Geometry: final body of the model. Coordinates: model frame, mm. Face numbers are marked on the shaded views. A direction names the side the tool comes from. Round coordinates to 2 decimals unless told otherwise and drop trailing zeros. Order: outer loops, then holes, each group sorted by start corner. A loop starts at its lowest first (then second) coordinate and runs counter-clockwise, first axis right, second up. Notation, with made-up numbers: (35.5, 32.25) - (64.5, 32.25) arc R23 ccw to (64.5, 63.25) - close; hole circle Ø9 at (-22.75, 68.5). An arc over 180 degrees is marked (long way). Put each result on its own line as item: value. Start each with the question number.
(1) Section B-B (y = 2.2). Output: boundary loops of the cut face in (x, z).
(2) Material intervals for L1, parallel to X at y = 2.35, z = 6; L2, parallel to X at y = 0.9, z = 6; L3, parallel to Z at x = 1, y = 2.1, sorted ascending. Write a range as [from, to].
(3) Pin query (flat end, axial travel): P1, Ø6, axis at x = -1.5, z = 1, coming from the +Y side; P2, Ø0.5, axis at y = 1.5, z = 6.5, coming from the +X side; P3, Ø2.5, axis at x = 1.25, z = 6, coming from the -Y side. Return the tip coordinate at first contact, or that it passes through.
(4) Access query for the marked faces 1, 2, 3, 4 and 5. Directions: +Z, -Z, +X, -X, +Y, -Y. A direction counts if a zero-diameter tool reaches every point of the face in a straight line with its end or side. Return the directions, or none.
(5) Section C-C (z = 6). Output: boundary loops of the cut face in (x, y).
(6) Pull-direction query (X, two-part tool) for the marked faces 6, 7 and 8; classes: released by +X, released by -X, zero draft, split by the parting line, or undercut.
(7) Section D-D (z = 2.5). Output: boundary loops of the cut face in (x, y).
(8) Section A-A (x = 1.25). Output: boundary loops of the cut face in (y, z).
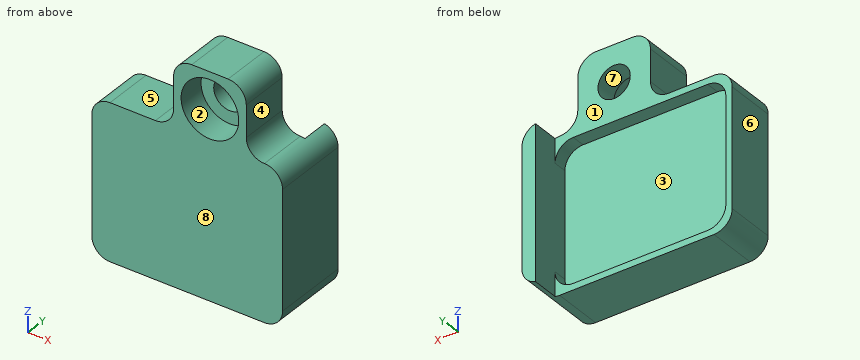
from build123d import *

# Parameters (mm, degrees)
SKETCH1_W                                      = 10.5
SKETCH1_H                                      = 8.5
EXTRUDE1_DEPTH                                 = 4.25
SKETCH3_W                                      = 9.75
SKETCH3_H                                      = 8.5
EXTRUDE4_DEPTH                                 = 1.5
SKETCH4_W                                      = 9.4
SKETCH4_H                                      = 7.8
EXTRUDE5_DEPTH                                 = 0.75
SKETCH5_W                                      = 4
SKETCH5_H                                      = 2.75
EXTRUDE6_DEPTH                                 = 3.75
CBORE_FOR_0_SOCKET_HEAD_CAP_SCREW1_D           = 1.778
CBORE_FOR_0_SOCKET_HEAD_CAP_SCREW1_CBORE_D     = 3.175
CBORE_FOR_0_SOCKET_HEAD_CAP_SCREW1_CBORE_DEPTH = 1.524
FILLET1_R                                      = 1


with BuildPart() as part:
    # Sketch1 → Extrude1 (new body)
    with BuildSketch(Plane(origin=(0, 0, 0), x_dir=(1, 0, 0), z_dir=(0, 1, 0))):
        Rectangle(SKETCH1_W, SKETCH1_H)
    extrude(amount=EXTRUDE1_DEPTH)

    # Sketch3 → Extrude4 (cut)
    with BuildSketch(Plane(origin=(0, 4.25, 0), x_dir=(1, 0, 0), z_dir=(0, 1, 0))):
        with Locations((-0.375, 0)):
            Rectangle(SKETCH3_W, SKETCH3_H)
    extrude(amount=-EXTRUDE4_DEPTH, mode=Mode.SUBTRACT)

    # Sketch4 → Extrude5 (cut)
    with BuildSketch(Plane(origin=(0, 2.75, 0), x_dir=(1, 0, 0), z_dir=(0, 1, 0))):
        with Locations((-0.2, 0)):
            Rectangle(SKETCH4_W, SKETCH4_H)
    extrude(amount=-EXTRUDE5_DEPTH, mode=Mode.SUBTRACT)

    # Sketch5 → Extrude6 (add)
    with BuildSketch(Plane.XY.offset(4.25)):
        with Locations((1.25, 1.375)):
            Rectangle(SKETCH5_W, SKETCH5_H)
    extrude(amount=EXTRUDE6_DEPTH)

    # CBORE for #0 Socket Head Cap Screw1 (through all)
    with Locations(Plane(origin=(1.25, 0, 6), x_dir=(0, 0, -1), z_dir=(0, -1, 0))):
        with Locations((0, 0)):
            CounterBoreHole(CBORE_FOR_0_SOCKET_HEAD_CAP_SCREW1_D / 2, CBORE_FOR_0_SOCKET_HEAD_CAP_SCREW1_CBORE_D / 2, CBORE_FOR_0_SOCKET_HEAD_CAP_SCREW1_CBORE_DEPTH)

    # Fillet1
    # the kernel refuses this fillet: 1 mm, written as the material it adds along each edge
    with BuildSketch(Plane(origin=(3.25, 2.75, 4.25), x_dir=(0, 0, 1), z_dir=(0, -1, 0))) as fillet1_piece_1:
        with BuildLine():
            CenterArc((FILLET1_R, -FILLET1_R), FILLET1_R, 90, 90)
            Line((0, -FILLET1_R), (0, 0))
            Line((0, 0), (FILLET1_R, 0))
        make_face()
    extrude(amount=2.75)
    with BuildSketch(Plane(origin=(-0.75, 0, 4.25), x_dir=(-1, 0, 0), z_dir=(0, 1, 0))) as fillet1_piece_2:
        with BuildLine():
            CenterArc((FILLET1_R, FILLET1_R), FILLET1_R, 180, 90)
            Line((0, FILLET1_R), (0, 0))
            Line((0, 0), (FILLET1_R, 0))
        make_face()
    extrude(amount=2.75)
    with BuildSketch(Plane(origin=(4.5, 2.75, -3.9), x_dir=(0, 0, 1), z_dir=(0, -1, 0)), Plane(origin=(-4.9, 2.75, -3.9), x_dir=(1, 0, 0), z_dir=(0, -1, 0)), Plane(origin=(-4.9, 2.75, 3.9), x_dir=(0, 0, -1), z_dir=(0, -1, 0))) as fillet1_piece_3:
        with BuildLine():
            CenterArc((FILLET1_R, FILLET1_R), FILLET1_R, 180, 90)
            Line((0, FILLET1_R), (0, 0))
            Line((0, 0), (FILLET1_R, 0))
        make_face()
    extrude(amount=0.75)
    with BuildSketch(Plane(origin=(4.5, 2.75, 3.9), x_dir=(0, 0, -1), z_dir=(0, -1, 0))) as fillet1_piece_4:
        with BuildLine():
            CenterArc((FILLET1_R, -FILLET1_R), FILLET1_R, 90, 90)
            Line((0, -FILLET1_R), (0, 0))
            Line((0, 0), (FILLET1_R, 0))
        make_face()
    extrude(amount=0.75)
    # the kernel refuses this fillet: 1 mm, written as the material it takes off along each edge
    with BuildSketch(Plane(origin=(5.25, -2.5, -4.25), x_dir=(-1, 0, 0), z_dir=(0, 1, 0)), Plane(origin=(5.25, -2.5, 4.25), x_dir=(0, 0, -1), z_dir=(0, 1, 0))) as fillet1_2_piece_1:
        with BuildLine():
            CenterArc((FILLET1_R, FILLET1_R), FILLET1_R, 180, 90)
            Line((0, FILLET1_R), (0, 0))
            Line((0, 0), (FILLET1_R, 0))
        make_face()
    extrude(amount=9.25, mode=Mode.SUBTRACT)
    with BuildSketch(Plane(origin=(3.25, 5.25, 8), x_dir=(0, 0, -1), z_dir=(0, -1, 0))) as fillet1_2_piece_2:
        with BuildLine():
            CenterArc((FILLET1_R, -FILLET1_R), FILLET1_R, 90, 90)
            Line((0, -FILLET1_R), (0, 0))
            Line((0, 0), (FILLET1_R, 0))
        make_face()
    extrude(amount=7.75, mode=Mode.SUBTRACT)
    with BuildSketch(Plane(origin=(-0.75, -2.5, 8), x_dir=(1, 0, 0), z_dir=(0, 1, 0)), Plane(origin=(-5.25, -2.5, -4.25), x_dir=(0, 0, 1), z_dir=(0, 1, 0)), Plane(origin=(-5.25, -2.5, 4.25), x_dir=(1, 0, 0), z_dir=(0, 1, 0))) as fillet1_2_piece_3:
        with BuildLine():
            CenterArc((FILLET1_R, FILLET1_R), FILLET1_R, 180, 90)
            Line((0, FILLET1_R), (0, 0))
            Line((0, 0), (FILLET1_R, 0))
        make_face()
    extrude(amount=7.75, mode=Mode.SUBTRACT)


solid = part.part
Checks:
1. outline: (-5.25, -3.25) arc R1 ccw to (-4.25, -4.25) - (4.25, -4.25) arc R1 ccw to (5.25, -3.25) - (5.25, 3.25) arc R1 ccw to (4.25, 4.25) arc R1 cw to (3.25, 5.25) - (3.25, 7) arc R1 ccw to (2.25, 8) - (0.25, 8) arc R1 ccw to (-0.75, 7) - (-0.75, 5.25) arc R1 cw to (-1.75, 4.25) - (-4.25, 4.25) arc R1 ccw to (-5.25, 3.25) - close; hole (-4.9, -2.9) arc R1 ccw to (-3.9, -3.9) - (3.5, -3.9) arc R1 ccw to (4.5, -2.9) - (4.5, 2.9) arc R1 ccw to (3.5, 3.9) - (-3.9, 3.9) arc R1 ccw to (-4.9, 2.9) - close; hole circle Ø1.78 at (1.25, 6)
2. L1: x = [-0.75, 0.36], [2.14, 3.25]
2. L2: x = [-0.75, -0.34], [2.84, 3.25]
2. L3: z = [-4.25, -3.9], [3.9, 5.15], [6.85, 8]
3. P1: stops at y = 2.75
3. P2: stops at x = 3.25
3. P3: stops at y = 1.52
4. face 1: +Z, -Z, -X, +Y
4. face 2: -Y
4. face 3: +Y
4. face 4: +Z, +X, +Y, -Y
4. face 5: +Z, -X, +Y, -Y
5. outline: (-0.75, 0) - (-0.34, 0) - (-0.34, 1.52) - (0.36, 1.52) - (0.36, 2.75) - (-0.75, 2.75) - close; (2.14, 1.52) - (2.84, 1.52) - (2.84, 0) - (3.25, 0) - (3.25, 2.75) - (2.14, 2.75) - close
6. face 6: released by -X
6. face 7: undercut
6. face 8: zero draft
7. outline: (-5.25, 0) - (5.25, 0) - (5.25, 4.25) - (4.5, 4.25) - (4.5, 2) - (-4.9, 2) - (-4.9, 2.75) - (-5.25, 2.75) - close
8. outline: (0, -4.25) - (2.75, -4.25) - (2.75, -3.9) - (2, -3.9) - (2, 3.9) - (2.75, 3.9) - (2.75, 5.11) - (1.52, 5.11) - (1.52, 4.41) - (0, 4.41) - close; (0, 7.59) - (1.52, 7.59) - (1.52, 6.89) - (2.75, 6.89) - (2.75, 8) - (0, 8) - close
